Here's the drawing with two shaded views (mm, measured from the low corner). I have some questions. Round coordinates to 2 decimals unless told otherwise and drop trailing zeros. Loops run counter-clockwise (first coordinate to the right, second up) from the corner with the lowest first, then second, coordinate; pieces in that order, holes last.
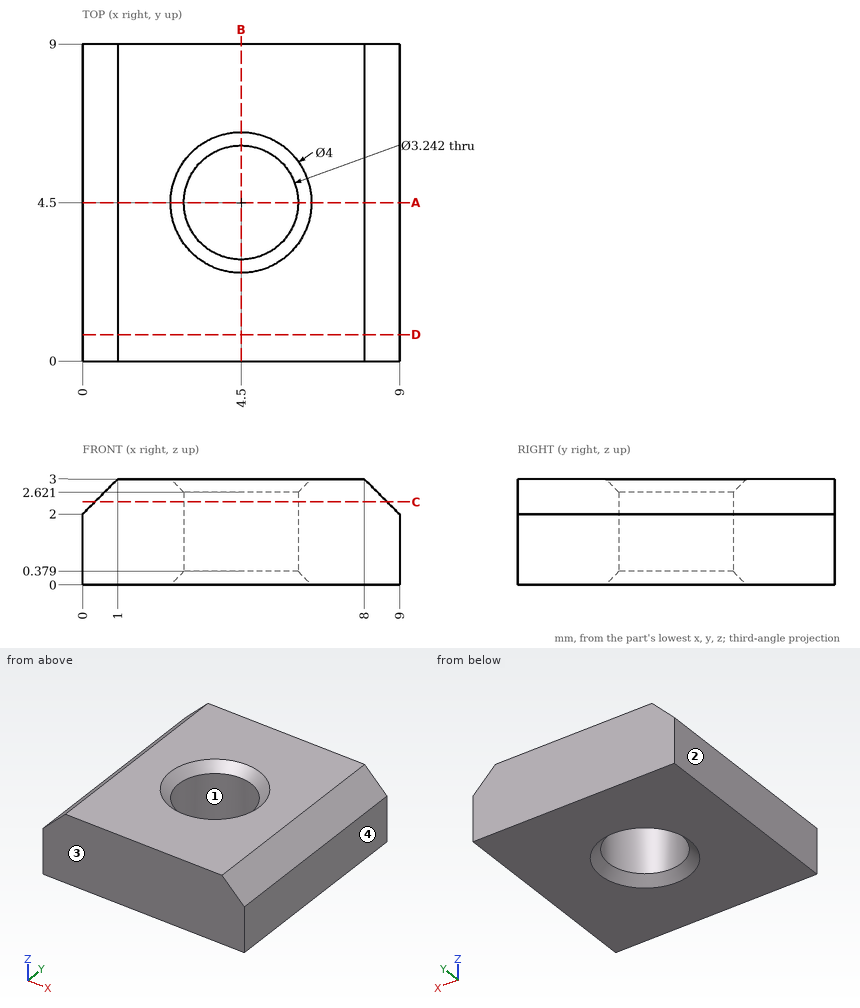
Item 1: If we section it at C-C, the plane z = 2.35: Please give me the cut outline in (x, y).
Results list:
outline: (0.35, 0) - (8.65, 0) - (8.65, 9) - (0.35, 9) - close; hole circle Ø3.24 at (4.5, 4.5)
Item 2: If I drill on line 1 along X through (y, z) = (4.5, 1.1); line 2 along Z through (x, y) = (8.5, 5); line 3 along Y through (x, z) = (3.25, 2), over which ranges is the centre line in solid material (lowest first)?
Results list:
line 1: x = 0 to 2.88, 6.12 to 9
line 2: z = 0 to 2.5
line 3: y = 0 to 3.47, 5.53 to 9
Item 3: If we section it at A-A, the plane y = 4.5: Please give me the cut outline in (x, z), then the cut area to 3 significant figures.
Results list:
outline: (0, 0) - (2.5, 0) - (2.88, 0.38) - (2.88, 2.62) - (2.5, 3) - (1, 3) - (0, 2) - close; (6.12, 0.38) - (6.5, 0) - (9, 0) - (9, 2) - (8, 3) - (6.5, 3) - (6.12, 2.62) - close
area: 16.0 mm2
Item 4: If we section it at B-B, the plane x = 4.5: Please give me the cut outline in (y, z), then the cut area to 3 significant figures.
Results list:
outline: (0, 0) - (2.5, 0) - (2.88, 0.38) - (2.88, 2.62) - (2.5, 3) - (0, 3) - close; (6.12, 0.38) - (6.5, 0) - (9, 0) - (9, 3) - (6.5, 3) - (6.12, 2.62) - close
area: 17.0 mm2
Item 5: Will this pin go through, and if not, where does the flat tip stop? pin 1 (3 mm diameter, centred on x = 4.5, y = 4.5, fed in from +Z).
Results list:
pin 1: passes through
Item 6: We'd pull the mould along X, two halves only. Please class the marked faces 1, 2, 3 and 4: released by +X, released by -X, zero draft, split by the parting line, or undercut.
Results list:
face 1: undercut
face 2: released by -X
face 3: zero draft
face 4: released by +X
Item 7: If we section it at D-D, the plane y = 0.75: Please give me the cut outline in (x, z), then the cut area to 3 significant figures.
Results list:
outline: (0, 0) - (9, 0) - (9, 2) - (8, 3) - (1, 3) - (0, 2) - close
area: 26.0 mm2
